Check sheet for the modelled part. Datum: model origin and axes. Units: mm. A direction names the side the tool comes from. Round coordinates to 2 decimals unless told otherwise and drop trailing zeros. Answer as a JSON object with one key per item and string values. Group by question number.
Item 1: Set-up check for faces 4 (the flat face through (25.4, 0, 14)), 5 (the flat face through (13, 7.938, -5)), 6 (the cylindrical face through (3.153, -0.767, 1.314)), 7 (the cylindrical face through (16, 16, 15)), 8 (the flat face through (6.096, 22.2, 14.7)): record each of +Z, -Z, +X, -X, +Y, -Y from which the full face is reachable in a straight line by a thin tool's end or side.
Item 2: Thickness scan on line 1 (Y direction, x = 3.25, z = 16.5); line 2 (Z direction, x = 15, y = -19.05) (3 decimals); line 3 (X direction, y = 0.5, z = 3.5). Record the ranges inside material, lowest first.
Item 3: Sectioned sample at A-A on z = 5. Count the separate pieces of the cut face and the enclosed holes in it, plus the area to 3 significant figures.
Item 4: Gauge pin test, flat ends, axial feed: P1, Ø9.5, axis at x = 15, z = -6.5, coming from the -Y side; P2, Ø3, axis at y = -17, z = 17, coming from the -X side. Record the tip position at first contact, or that the pin passes through.
Item 5: Release check for a two-part mould opening along X. For faces 1 (the conical face through (19.369, -0.019, 10.792)), 2 (the cylindrical face through (15.883, -15.878, 15.735)), 3 (the flat face through (15.875, 0, 16)) record: pulls with the +X half, pulls with the -X half, needs draft (parallel to the pull), parting line crosses it, or undercut.
```python
from build123d import *

# Parameters (mm, degrees)
F0_R           = 4.7625
F1_DEPTH       = 25.4
F2_D           = 6.35
F2_CBORE_D     = 9.525
F2_CBORE_DEPTH = 6.096
F3_DEPTH       = 15.875
F4_R           = 3.175
F6_D           = 5.1054
F6_DEPTH       = 25.4
F6_TIP         = 1.5338169022
F7_D           = 5.1054
F7_DEPTH       = 19.05
F7_TIP         = 1.5338169022


with BuildPart() as f1:
    # F0 (on Right) → F1 (new body)
    with BuildSketch(Plane.YZ):
        with BuildLine():
            Line((-7.9375, -9.525), (0, -9.525))
            Line((0, -9.525), (7.9375, -9.525))
            Line((7.9375, -9.525), (7.9375, -0.79375))
            ThreePointArc((7.9375, -0.79375), (7.3762339924, 0.5612660076), (8.73125, 0))
            Line((8.73125, 0), (30.1625, 0))
            Line((30.1625, 0), (30.1625, 28.575))
            Line((30.1625, 28.575), (0, 28.575))
            Line((0, 28.575), (-30.1625, 28.575))
            Line((-30.1625, 28.575), (-30.1625, 0))
            Line((-30.1625, 0), (-8.73125, 0))
            ThreePointArc((-8.73125, 0), (-7.3762339924, 0.5612660076), (-7.9375, -0.79375))
            Line((-7.9375, -0.79375), (-7.9375, -9.525))
        make_face()
        with Locations((0, 15.875)):
            Circle(F0_R, mode=Mode.SUBTRACT)
        with Locations((0, 15.875)):
            Circle(F0_R)
    extrude(amount=F1_DEPTH)

    # F2 (through all)
    with Locations(Plane(origin=(0, 0, 0), x_dir=(0, 1, 0), z_dir=(-1, 0, 0))):
        with Locations((-19.05, -15.875), (19.05, -15.875)):
            CounterBoreHole(F2_D / 2, F2_CBORE_D / 2, F2_CBORE_DEPTH)

    # F0 (on Right) → F3 (cut)
    with BuildSketch(Plane.YZ):
        with Locations((0, 15.875)):
            Circle(F0_R)
    extrude(amount=F3_DEPTH, mode=Mode.SUBTRACT)

    # F4
    f4_edges = [f1.edges().sort_by_distance(p)[0] for p in [
        (12.7, -30.1625, 28.575),
        (12.7, 30.1625, 28.575),
        (0, 0, 28.575),
        (0, -30.1625, 14.2875),
        (0, 30.1625, 14.2875),
    ]]
    fillet(f4_edges, radius=F4_R)

    # F6
    with Locations(Plane(origin=(0, 0, -9.525), x_dir=(1, 0, 0), z_dir=(0, 0, -1))):
        with Locations((5.588, 0)):
            Hole(F6_D / 2, depth=F6_DEPTH)
            with Locations((0, 0, -(F6_DEPTH + F6_TIP / 2))):  # 118° drill point
                Cone(0, F6_D / 2, F6_TIP, mode=Mode.SUBTRACT)

    # F7
    with Locations(Plane(origin=(0, 0, -9.525), x_dir=(1, 0, 0), z_dir=(0, 0, -1))):
        with Locations((19.812, 0)):
            Hole(F7_D / 2, depth=F7_DEPTH)
            with Locations((0, 0, -(F7_DEPTH + F7_TIP / 2))):  # 118° drill point
                Cone(0, F7_D / 2, F7_TIP, mode=Mode.SUBTRACT)


solid = f1.part
```
Completed:
{
 "1": {"face 4": "+Z, -Z, +X, +Y, -Y", "face 5": "-Z, +X, -X, +Y", "face 6": "-Z", "face 7": "+X, -X", "face 8": "-X"},
 "2": {"line 1": "-30.16 to -23.77, -14.33 to -4.72, 4.72 to 14.33, 23.77 to 30.16", "line 2": "0 to 12.7, 19.05 to 28.575", "line 3": "0 to 3.08, 8.09 to 17.31, 22.32 to 25.4"},
 "3": {"separate pieces": "1", "enclosed holes": "2", "area": "1,490 mm²"},
 "4": {"P1": "y = -7.94", "P2": "x = 6.1"},
 "5": {"face 1": "undercut", "face 2": "needs draft", "face 3": "pulls with the -X half"}
}
